Part model, mm, in its own coordinate system. A direction names the side the tool comes from. Coordinates: 2 decimals unless noted, no trailing zeros. Loops run counter-clockwise (first coordinate to the right, second up) from the corner with the lowest first, then second, coordinate; pieces in that order, holes last. Notation, with made-up numbers: M 55,16.5 L 68,16.5 A24 cw 68,52.5 Z; hole C 33.25,28.25 d5. An arc over 180 degrees is marked long. Answer as a JSON object with one key per item and string values. Group by question number.
1. Mould opens along Y. For faces 1 (the face through (3518.284, 1059, 3)), 2 (the face through (3538.336, 1075, 3)), 3 (the face through (3515, 1055.749, 3)), 4 (the face through (3529.214, 1101.668, 2.958)) say: released by +Y, released by -Y, zero draft, split by the parting line, or undercut.
2. Drill centre lines: L1, parallel to X at y = 1073.5, z = 2.4; L2, parallel to X at y = 1068.5, z = 3.35; L3, parallel to X at y = 1070, z = 1.65. Where is each one in solid material? Low to high.
3. Drop flat-ended pins along their axis: pin 1 Ø3 at (x, z) = (3497.5, 3) entering from -Y; pin 2 Ø1.8 at (y, z) = (1073.5, 2) entering from -X; pin 3 Ø3 at (x, z) = (3515.5, 3) entering from +Y. Give the stop position or say it passes through.
4. Saw through at C-C on x = 3517. Write the cut outline in (y, z), then the cut area to 3 significant figures.
5. Saw through at D-D on x = 3501.5. Write the cut outline in (y, z), then the cut area to 3 significant figures.
6. Saw through at B-B on y = 1070.5. Write the cut outline in (x, z), then the cut area to 3 significant figures.
7. 3-axis set-ups, long thin cutter, end or side, ignore diameter. For faces 5 (the face through (3562, 1061.749, 3)), 6 (the face through (3500, 1061.749, 3)), 7 (the face through (3534, 1061.749, 3)), 8 (the face through (3531.336, 1069, 3)): which of +Z, -Z, +X, -X, +Y, -Y reach the whole face in a straight line?
from build123d import *

# Parameters (mm, degrees)
MODEL_W             = 6
MODEL_H             = 6
BOSS_EXTRUDE1_DEPTH = 6


with BuildPart() as part:
    # Model → Boss-Extrude1 (new body)
    with BuildSketch(Plane.XY):
        with BuildLine():
            Line((3550.284318909, 1061.748947436), (3550.284318909, 1055.748947436))
            Line((3550.284318909, 1055.748947436), (3556.284318909, 1055.748947436))
            Line((3556.284318909, 1055.748947436), (3556.284318909, 1061.748947436))
            Line((3556.284318909, 1061.748947436), (3568.264255366, 1061.748947436))
            ThreePointArc((3568.264255366, 1061.748947436), (3528.335683937, 1101.677518865), (3488.407112509, 1061.748947436))
            Line((3488.407112509, 1061.748947436), (3512.284318909, 1061.748947436))
            Line((3512.284318909, 1061.748947436), (3512.284318909, 1055.748947436))
            Line((3512.284318909, 1055.748947436), (3518.284318909, 1055.748947436))
            Line((3518.284318909, 1055.748947436), (3518.284318909, 1061.748947436))
            Line((3518.284318909, 1061.748947436), (3550.284318909, 1061.748947436))
        make_face()
        with Locations((3541.335683937, 1074.748947436)):
            Rectangle(MODEL_W, MODEL_H, mode=Mode.SUBTRACT)
        with Locations((3515.335683937, 1074.748947436)):
            Rectangle(MODEL_W, MODEL_H, mode=Mode.SUBTRACT)
        with Locations((3528.335683937, 1080.748947436)):
            Rectangle(MODEL_W, MODEL_H, mode=Mode.SUBTRACT)
        with Locations((3528.335683937, 1068.57340627)):
            Rectangle(MODEL_W, MODEL_H, mode=Mode.SUBTRACT)
    extrude(amount=BOSS_EXTRUDE1_DEPTH)


solid = part.part
Outcome:
{
 "1": {"face 1": "zero draft", "face 2": "undercut", "face 3": "released by -Y", "face 4": "released by +Y"},
 "2": {"L1": "x = 3490.18 to 3512.34, 3518.34 to 3538.34, 3544.34 to 3566.5", "L2": "x = 3488.98 to 3525.34, 3531.34 to 3567.69", "L3": "x = 3489.27 to 3525.34, 3531.34 to 3567.4"},
 "3": {"pin 1": "stops at y = 1061.75", "pin 2": "stops at x = 3489.91", "pin 3": "stops at y = 1100.03"},
 "4": {"outline": "M 1055.75,0 L 1071.75,0 L 1071.75,6 L 1055.75,6 Z; M 1077.75,0 L 1100.03,0 L 1100.03,6 L 1077.75,6 Z", "area": "230 mm²"},
 "5": {"outline": "M 1061.75,0 L 1091.31,0 L 1091.31,6 L 1061.75,6 Z", "area": "177 mm²"},
 "6": {"outline": "M 3489.38,0 L 3525.34,0 L 3525.34,6 L 3489.38,6 Z; M 3531.34,0 L 3567.29,0 L 3567.29,6 L 3531.34,6 Z", "area": "431 mm²"},
 "7": {"face 5": "+Z, -Z, +X, -Y", "face 6": "+Z, -Z, -X, -Y", "face 7": "+Z, -Z, -Y", "face 8": "+Z, -Z"}
}
